Geometry check sheet. Reference: the model listing, model coordinates, mm. Face numbers are marked on the shaded views. A direction names the side the tool comes from. Give positions to 0.01 mm unless a question says otherwise; leave off trailing zeros. Write each loop counter-clockwise with the first axis right and the second up, starting at its lowest first coordinate (ties: lowest second). Pieces come first, ordered by that corner, then holes. Notation, with made-up numbers: (25, -31.5) -> (34, -31.5) arc R21 cw to (34, -16.5) -> close; hole circle Ø3 at (25, -24). An arc over 180 degrees is marked (long way). Use a Markdown table: item, result. Add a question column.
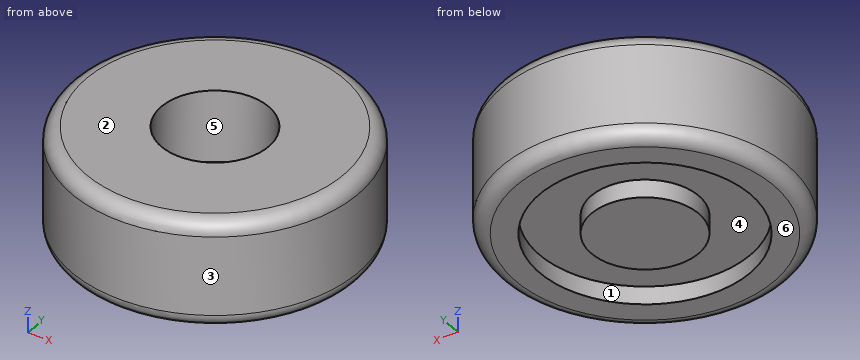
from build123d import *

# Parameters (mm, degrees)
SKETCH1_R           = 101.6
SKETCH1_R_2         = 38.1
BOSS_EXTRUDE7_DEPTH = 76.2
SKETCH1_11_R        = 38.1
BOSS_EXTRUDE9_DEPTH = 25.4
FILLET1_R           = 10.16
SKETCH2_R           = 74.820465974
SKETCH2_R_2         = 38.1
CUT_EXTRUDE1_DEPTH  = 12.7


with BuildPart() as part:
    # Sketch1 → Boss-Extrude7 (new body)
    with BuildSketch(Plane.XY):
        with Locations(Location((0, 0, 0), (0, 0, 180))):
            Circle(SKETCH1_R)
        with Locations(Location((0, 0, 0), (0, 0, 180))):
            Circle(SKETCH1_R_2, mode=Mode.SUBTRACT)
    extrude(amount=BOSS_EXTRUDE7_DEPTH)

    # Sketch1_11 → Boss-Extrude9 (add)
    with BuildSketch(Plane.XY):
        with Locations(Location((0, 0, 0), (0, 0, 180))):
            Circle(SKETCH1_11_R)
    extrude(amount=BOSS_EXTRUDE9_DEPTH)

    # Fillet1
    fillet1_edges = [part.edges().sort_by_distance(p)[0] for p in [
        (101.6, 0, 76.2),
        (101.6, 0, 0),
    ]]
    fillet(fillet1_edges, radius=FILLET1_R)

    # Sketch2 → Cut-Extrude1 (cut)
    with BuildSketch(Plane(origin=(0, 0, 0), x_dir=(-1, 0, 0), z_dir=(0, 0, -1))):
        Circle(SKETCH2_R)
        Circle(SKETCH2_R_2, mode=Mode.SUBTRACT)
    extrude(amount=-CUT_EXTRUDE1_DEPTH, mode=Mode.SUBTRACT)


solid = part.part
1) Sectioned sample at A-A, the plane z = 57. Enter the section's corners in (x, y).
2) Material ranges on probe 1 along Y at (x, z) = (0, 63.5); probe 2 along X at (y, z) = (13, 4.5); probe 3 along Y at (x, z) = (-23, 3.5), recorded low to high. Write a range as [from, to].
3) Tool access check on the marked faces 4, 5 and 6. Record the directions out of +Z, -Z, +X, -X, +Y, -Y that give a thin tool (end or side, any length) a straight path to the whole face; none if there is none.
4) Draft check along X on the marked faces 1, 2 and 3. Enter one of: +X half, -X half, draft (parallel to the pull), parting line (faces both ways), or undercut.
5) Gauge pin test, flat ends, axial feed: P1, Ø5, axis at x = 7, z = 60, coming from the -Y side; P2, Ø12, axis at x = 39, z = 32.5, coming from the +Y side; P3, Ø6, axis at x = -6.5, z = 65.5, coming from the +Y side. Record the tip position at first contact, or that the pin passes through.
6) Sectioned sample at B-B, the plane y = 0. Enter the section's corners in (x, z).
7) Sectioned sample at D-D, the plane z = 70. Enter the section's corners in (x, y), and give its area (3 significant figures).
Check values:
| question | item | result |
|---|---|---|
| 1 | outline | circle Ø203.2 at (0, 0); hole circle Ø76.2 at (0, 0) |
| 2 | probe 1 | [-101.6, -38.1], [38.1, 101.6] |
| 2 | probe 2 | [-99.03, -73.68], [-35.81, 35.81], [73.68, 99.03] |
| 2 | probe 3 | [-96.41, -71.2], [-30.37, 30.37], [71.2, 96.41] |
| 3 | face 4 | -Z |
| 3 | face 5 | +Z |
| 3 | face 6 | -Z, +X, -X, +Y, -Y |
| 4 | face 1 | undercut |
| 4 | face 2 | draft |
| 4 | face 3 | parting line |
| 5 | P1 | y = -101.5 |
| 5 | P2 | y = 96.09 |
| 5 | P3 | y = 101.54 |
| 6 | outline | (-101.6, 10.16) arc R10.16 ccw to (-91.44, 0) -> (-74.82, 0) -> (-74.82, 12.7) -> (-38.1, 12.7) -> (-38.1, 0) -> (38.1, 0) -> (38.1, 12.7) -> (74.82, 12.7) -> (74.82, 0) -> (91.44, 0) arc R10.16 ccw to (101.6, 10.16) -> (101.6, 66.04) arc R10.16 ccw to (91.44, 76.2) -> (38.1, 76.2) -> (38.1, 25.4) -> (-38.1, 25.4) -> (-38.1, 76.2) -> (-91.44, 76.2) arc R10.16 ccw to (-101.6, 66.04) -> close |
| 7 | outline | circle Ø201.59 at (0, 0); hole circle Ø76.2 at (0, 0) |
| 7 | area | 27,400 mm² |
